from build123d import *

# Parameters (mm, degrees)
F0_W     = 381
F0_H     = 152.4
F1_DEPTH = 12.7
F3_D     = 9.525
F4_D     = 9.525
F5_W     = 25.4
F5_H     = 25.4
F6_DEPTH = 12.7


with BuildPart() as f1:
    # F0 (on Top) → F1 (new body)
    with BuildSketch(Plane.XY):
        Rectangle(F0_W, F0_H)
    extrude(amount=F1_DEPTH)

    # F3 (through all)
    with Locations(Plane.XY.offset(12.7)):
        with Locations((-165.1, 50.8)):
            Hole(F3_D / 2)

    # F4 (through all)
    with Locations(Plane.XY.offset(12.7)):
        with Locations((-95.25, 50.8), (0, 50.8), (95.25, 50.8), (165.1, 50.8), (128.5875, 0), (50.8, 0), (-50.8, 0), (-128.5875, 0), (-165.1, -50.8), (-95.25, -50.8), (0, -50.8), (95.25, -50.8), (165.1, -50.8)):
            Hole(F4_D / 2)

    # F5 (on face) → F6 (cut)
    with BuildSketch(Plane.XY.offset(12.7)):
        with Locations((127, 0)):
            Rectangle(F5_W, F5_H)
    extrude(amount=-F6_DEPTH, mode=Mode.SUBTRACT)


solid = f1.part
Part model, mm, in its own coordinate system. A direction names the side the tool comes from. Give positions to 0.01 mm unless a question says otherwise; leave off trailing zeros. Order: outer loops, then holes, each group sorted by start corner. A loop starts at its lowest first (then second) coordinate and runs counter-clockwise, first axis right, second up. Notation, with made-up numbers: (4, -29.75) - (23, -29.75) arc R19 cw to (23, 4.25) - close; hole circle Ø2 at (42.25, -7.5). An arc over 180 degrees is marked (long way). Use a Markdown table: item, result.
1) Flat gauge pin, fed straight in: P1, Ø5.5, axis at x = -128.59, y = 0, coming from the -Z side. Where does the tip first touch, or does it go through?
Checked values:
| item | result |
|---|---|
| P1 | through |
2) 3-axis set-ups, long thin cutter, end or side, ignore diameter. For faces 1 (the flat face through (139.7, 0, 6)), 2 (the flat face through (-3, 1, 12.7)): which of +Z, -Z, +X, -X, +Y, -Y reach the whole face in a straight line?
Checked values:
| item | result |
|---|---|
| face 1 | +Z, -Z |
| face 2 | +Z, +X, -X, +Y, -Y |
3) Probe L1, parallel to Y at x = 95.25, z = 8; L2, parallel to X at y = -9, z = 3.75; L3, parallel to X at y = -51.5, z = 11. List the from-to ranges inside material, lowest first. Write a range as from..to.
Checked values:
| item | result |
|---|---|
| L1 | -76.2..-55.56, -46.04..46.04, 55.56..76.2 |
| L2 | -190.5..114.3, 139.7..190.5 |
| L3 | -190.5..-169.81, -160.39..-99.96, -90.54..-4.71, 4.71..90.54, 99.96..160.39, 169.81..190.5 |
4) Saw through at A-A on x = -50.8. List the corners of the cut face in (y, z).
Checked values:
| item | result |
|---|---|
| outline | (-76.2, 0) - (-4.76, 0) - (-4.76, 12.7) - (-76.2, 12.7) - close; (4.76, 0) - (76.2, 0) - (76.2, 12.7) - (4.76, 12.7) - close |
5) Two-plate mould, pull along X, no slides. Class faces 3 (the flat face through (127, 12.7, 6)), 4 (the flat face through (-3, -76.2, 6)), 5 (the flat face through (-190.5, -1, 6)): +X half, -X half, draft (parallel to the pull), parting line (faces both ways), or undercut.
Checked values:
| item | result |
|---|---|
| face 3 | undercut |
| face 4 | draft |
| face 5 | -X half |
6) Saw through at B-B on y = 50.8. List the corners of the cut face in (x, z).
Checked values:
| item | result |
|---|---|
| outline | (-190.5, 0) - (-169.86, 0) - (-169.86, 12.7) - (-190.5, 12.7) - close; (-160.34, 0) - (-100.01, 0) - (-100.01, 12.7) - (-160.34, 12.7) - close; (-90.49, 0) - (-4.76, 0) - (-4.76, 12.7) - (-90.49, 12.7) - close; (4.76, 0) - (90.49, 0) - (90.49, 12.7) - (4.76, 12.7) - close; (100.01, 0) - (160.34, 0) - (160.34, 12.7) - (100.01, 12.7) - close; (169.86, 0) - (190.5, 0) - (190.5, 12.7) - (169.86, 12.7) - close |
7) Saw through at C-C on x = 95.25. List the corners of the cut face in (y, z).
Checked values:
| item | result |
|---|---|
| outline | (-76.2, 0) - (-55.56, 0) - (-55.56, 12.7) - (-76.2, 12.7) - close; (-46.04, 0) - (46.04, 0) - (46.04, 12.7) - (-46.04, 12.7) - close; (55.56, 0) - (76.2, 0) - (76.2, 12.7) - (55.56, 12.7) - close |
